```python
from build123d import *

# Parameters (mm, degrees)
SKETCH5_R          = 12.7
CUT_EXTRUDE2_DEPTH = 49.864135621
SKETCH6_W          = 10.16
SKETCH6_H          = 10.16
CUT_EXTRUDE3_DEPTH = 6


with BuildPart() as part:
    # Sketch4 → Revolve4 (revolve)
    with BuildSketch(Plane(origin=(0, 0, 0), x_dir=(1, 0, 0), z_dir=(0, 1, 0))):
        with BuildLine():
            Line((-12, 18.706967285), (0, 18.706967285))
            Line((0, 18.706967285), (0, -18.706967285))
            Line((0, -18.706967285), (-12, -18.706967285))
            ThreePointArc((-12, -18.706967285), (-22.225, 0), (-12, 18.706967285))
        make_face()
    revolve(axis=Axis((0, 0, -17.487077089), (0, 0, 1)))

    # Sketch5 → Cut-Extrude2 (cut, through all)
    with BuildSketch(Plane.XY.offset(18.706967285)):
        with Locations(Location((0, 0, 0), (0, 0, 180))):
            Circle(SKETCH5_R)
    extrude(amount=-CUT_EXTRUDE2_DEPTH, mode=Mode.SUBTRACT)

    # Sketch6 → Cut-Extrude3 (cut)
    with BuildSketch(Plane(origin=(0, 22.225, 0), x_dir=(1, 0, 0), z_dir=(0, 1, 0))):
        Rectangle(SKETCH6_W, SKETCH6_H)
    cut_extrude3 = extrude(amount=-CUT_EXTRUDE3_DEPTH, mode=Mode.SUBTRACT)

    # Mirror1: Cut-Extrude3 across plane
    add(cut_extrude3.mirror(Plane.ZX), mode=Mode.SUBTRACT)


solid = part.part
```
Model file for the job. Use its own axes, mm. A direction names the side the tool comes from. Round coordinates to 2 decimals unless told otherwise and drop trailing zeros. Write each loop counter-clockwise with the first axis right and the second up, starting at its lowest first coordinate (ties: lowest second). Pieces come first, ordered by that corner, then holes. Notation, with made-up numbers: (8.25, 76.5) -> (46.25, 76.5) arc R26 ccw to (46.25, 107.5) -> close; hole circle Ø7 at (37, -17.5). An arc over 180 degrees is marked (long way). Answer as CSV lines item,"result".
1. Slice it at B-B, the plane z = -0.5. List the corners of the cut face in (x, y) (3 decimals).
Resolved:
outline,"(-5.08, -21.631) -> (-5.08, -16.225) -> (5.08, -16.225) -> (5.08, -21.631) arc R22.219 ccw to (5.08, 21.631) -> (5.08, 16.225) -> (-5.08, 16.225) -> (-5.08, 21.631) arc R22.219 ccw to start; hole circle Ø25.4 at (0, 0)"
2. Slice it at D-D, the plane y = 18. List the corners of the cut face in (x, z).
Resolved:
outline,"circle Ø26.07 at (0, 0); hole (-5.08, -5.08) -> (5.08, -5.08) -> (5.08, 5.08) -> (-5.08, 5.08) -> close"
3. Mould opens along Z. For faces 3 (the face through (5.08, 19, 0)), 4 (the face through (-5.86, 11.267, 0.255)) say: +Z half, -Z half, draft (parallel to the pull), parting line (faces both ways), or undercut.
Resolved:
face 3,"undercut"
face 4,"draft"
4. Pin check, flat tips, straight feed: pin 1 Ø3 at (y, z) = (-5.5, 9.5) entering from -X; pin 2 Ø3 at (y, z) = (15.5, -4.5) entering from -X; pin 3 Ø10 at (y, z) = (13.5, 10.5) entering from +X. Stop position of each tip, or through.
Resolved:
pin 1,"x = -20.1"
pin 2,"x = -16.72"
pin 3,"x = 18.64"
5. Slice it at C-C, the plane y = 0. List the corners of the cut face in (x, z) (3 decimals), plus the area to 3 significant figures.
Resolved:
outline,"(-12.7, -18.239) -> (-12.7, 18.239) arc R22.225 ccw to start; (12.7, -18.239) arc R22.225 ccw to (12.7, 18.239) -> close"
area,"488 mm²"
6. Drill centre lines: line 1 (Y direction, x = 0, z = -0.5) (3 decimals); line 2 (X direction, y = -18.5, z = 5); line 3 (Y direction, x = 1.5, z = -14.5). Where is each one in solid material? Low to high.
Resolved:
line 1,"-16.225 to -12.7, 12.7 to 16.225"
line 2,"-11.26 to -5.08, 5.08 to 11.26"
line 3,"-16.78 to -12.61, 12.61 to 16.78"
7. Tool access for faces 1 (the face through (-5.08, 19, 0)), 2 (the face through (0, -16.225, 0)): list every direction of +Z, -Z, +X, -X, +Y, -Y with a clear straight run to the whole face (end or side of a thin tool).
Resolved:
face 1,"+Y"
face 2,"-Y"
8. Slice it at A-A, the plane x = 0. List the corners of the cut face in (y, z) (3 decimals).
Resolved:
outline,"(-21.637, -5.08) arc R22.225 ccw to (-12.7, -18.239) -> (-12.7, 18.239) arc R22.225 ccw to (-21.637, 5.08) -> (-16.225, 5.08) -> (-16.225, -5.08) -> close; (12.7, -18.239) arc R22.225 ccw to (21.637, -5.08) -> (16.225, -5.08) -> (16.225, 5.08) -> (21.637, 5.08) arc R22.225 ccw to (12.7, 18.239) -> close"
